from build123d import *

# Parameters (mm, degrees)
SKETCH1_W           = 11
SKETCH1_H           = 15
BOSS_EXTRUDE1_DEPTH = 10
SKETCH3_R           = 3.4
CUT_EXTRUDE1_DEPTH  = 22.118712082
CUT_EXTRUDE2_DEPTH  = 22.118712082
FILLET1_R           = 1
SKETCH5_W           = 30.35499422
SKETCH5_H           = 5.878934171
SKETCH5_W_2         = 28.690297522
SKETCH5_H_2         = 3.597414723
CUT_EXTRUDE3_DEPTH  = 5
FILLET2_R           = 0.5


with BuildPart() as part:
    # Sketch1 → Boss-Extrude1 (new body)
    with BuildSketch(Plane(origin=(0, 0, 0), x_dir=(0, 0, -1), z_dir=(1, 0, 0))):
        with Locations((5.5, 7.5)):
            Rectangle(SKETCH1_W, SKETCH1_H)
    extrude(amount=BOSS_EXTRUDE1_DEPTH)

    # Sketch3 → Cut-Extrude1 (cut, through all)
    with BuildSketch(Plane.ZY):
        with Locations((-5.5, 7.5)):
            Circle(SKETCH3_R)
    extrude(amount=-CUT_EXTRUDE1_DEPTH, mode=Mode.SUBTRACT)

    # Sketch4 → Cut-Extrude2 (cut, through all)
    with BuildSketch(Plane.ZY):
        with BuildLine():
            Line((-8.5, 15), (-8.5, 13.5))
            ThreePointArc((-8.5, 13.5), (-8.792893219, 12.792893219), (-9.5, 12.5))
            Line((-9.5, 12.5), (-12.5, 12.5))
            Line((-12.5, 12.5), (-12.5, 2.5))
            Line((-12.5, 2.5), (-9.5, 2.5))
            ThreePointArc((-9.5, 2.5), (-8.792893219, 2.207106781), (-8.5, 1.5))
            Line((-8.5, 1.5), (-8.5, 0))
            Line((-8.5, 0), (-16.5, 0))
            Line((-16.5, 0), (-16.5, 15))
            Line((-16.5, 15), (-8.5, 15))
        make_face()
        with BuildLine():
            Line((-2.5, 1.5), (-2.5, 0))
            Line((-2.5, 0), (6, 0))
            Line((6, 0), (6, 15))
            Line((6, 15), (-2.5, 15))
            Line((-2.5, 15), (-2.5, 13.5))
            ThreePointArc((-2.5, 13.5), (-2.207106781, 12.792893219), (-1.5, 12.5))
            Line((-1.5, 12.5), (1.5, 12.5))
            Line((1.5, 12.5), (1.5, 2.5))
            Line((1.5, 2.5), (-1.5, 2.5))
            ThreePointArc((-1.5, 2.5), (-2.207106781, 2.207106781), (-2.5, 1.5))
        make_face()
    extrude(amount=-CUT_EXTRUDE2_DEPTH, mode=Mode.SUBTRACT)

    # Fillet1
    fillet1_edges = [part.edges().sort_by_distance(p)[0] for p in [
        (5, 12.5, -11),
        (5, 2.5, -11),
        (5, 0, -8.5),
        (5, 15, -8.5),
        (5, 15, -2.5),
        (5, 2.5, 0),
        (5, 12.5, 0),
        (5, 0, -2.5),
    ]]
    fillet(fillet1_edges, radius=FILLET1_R)

    # Sketch5 → Cut-Extrude3 (cut)
    with BuildSketch(Plane.ZY):
        with Locations((-1.883853424, 16.939467085)):
            Rectangle(SKETCH5_W, SKETCH5_H)
        with Locations((-4.752769967, -0.798707361)):
            Rectangle(SKETCH5_W_2, SKETCH5_H_2)
    extrude(amount=-CUT_EXTRUDE3_DEPTH, mode=Mode.SUBTRACT)

    # Fillet2
    fillet2_edges = [part.edges().sort_by_distance(p)[0] for p in [
        (2.5, 1, -8.5),
        (2.5, 1, -2.5),
        (2.5, 14, -8.5),
        (2.5, 14, -2.5),
    ]]
    fillet(fillet2_edges, radius=FILLET2_R - 0.0001)  # a hair under: the kernel refuses the full size


solid = part.part
CAD build for the part. Positions are in the model's coordinates, mm. A direction names the side the tool comes from. Round coordinates to 2 decimals unless told otherwise and drop trailing zeros. Loops run counter-clockwise (first coordinate to the right, second up) from the corner with the lowest first, then second, coordinate; pieces in that order, holes last. Notation, with made-up numbers: (77.5, 68.25) - (130.5, 68.25) arc R26 ccw to (130.5, 89.25) - close; hole circle Ø9 at (-3, 29). An arc over 180 degrees is marked (long way). Put each result on its own line as item: value.
1. Pin check, flat tips, straight feed: P1, Ø3, axis at x = 1, z = -7.5, coming from the +Y side; P2, Ø0.7, axis at y = 0.5, z = -6, coming from the -X side; P3, Ø4, axis at x = 2.5, z = -6.5, coming from the -Y side. Stop position of each tip, or through.
Geometry check:
P1: y = 14
P2: x = 5
P3: y = 1
2. Wall check: line 1 (Y direction, x = 3.75, z = -5.5); line 2 (Y direction, x = 5.5, z = -5.5); line 3 (Z direction, x = 5.75, y = 5.5). Give the ranges that are in metal, low to high.
Geometry check:
line 1: 1 to 4.1, 10.9 to 14
line 2: 0 to 4.1, 10.9 to 15
line 3: -11 to -8.25, -2.75 to 0
3. Two-plate mould, pull along Y, no slides. Class faces 1 (the cylindrical face through (5.07, 12.199, -0.285)), 2 (the cylindrical face through (4.93, 6.2, -2.36)), 3 (the cylindrical face through (5.07, 2.801, -10.715)), 4 (the flat face through (10, 4, -7)): released by +Y, released by -Y, zero draft, split by the parting line, or undercut.
Geometry check:
face 1: released by +Y
face 2: undercut
face 3: released by -Y
face 4: zero draft
4. Slice it at B-B on y = 7.5. List the corners of the cut face in (x, z).
Geometry check:
outline: (0, -11) - (10, -11) - (10, -8.9) - (0, -8.9) - close; (0, -2.1) - (10, -2.1) - (10, 0) - (0, 0) - close
5. Slice it at D-D on y = 9.75. List the corners of the cut face in (x, z).
Geometry check:
outline: (0, -11) - (10, -11) - (10, -8.05) - (0, -8.05) - close; (0, -2.95) - (10, -2.95) - (10, 0) - (0, 0) - close
6. 3-axis set-ups, long thin cutter, end or side, ignore diameter. For faces 5 (the flat face through (2, 14, -6)), 6 (the flat face through (2, 1, -6)), 7 (the cylindrical face through (4.93, 12.215, -10.699)): which of +Z, -Z, +X, -X, +Y, -Y reach the whole face in a straight line?
Geometry check:
face 5: +Z, -Z, -X, +Y
face 6: +Z, -Z, -X, -Y
face 7: -Z, +X, -X, +Y
7. Slice it at C-C on z = -5.5. List the corners of the cut face in (x, y).
Geometry check:
outline: (0, 1) - (5, 1) - (5, 0) - (10, 0) - (10, 4.1) - (0, 4.1) - close; (0, 10.9) - (10, 10.9) - (10, 15) - (5, 15) - (5, 14) - (0, 14) - close
